For this review, take the finished solid that the model builds, in its own axes (mm). Face numbers are marked on the shaded views. A direction names the side the tool comes from. Round coordinates to 2 decimals unless told otherwise and drop trailing zeros. Order: outer loops, then holes, each group sorted by start corner. A loop starts at its lowest first (then second) coordinate and runs counter-clockwise, first axis right, second up. Notation, with made-up numbers: (77.5, -18) - (81.5, -18) arc R29 cw to (81.5, 13) - close; hole circle Ø3 at (32, -1). An arc over 180 degrees is marked (long way). One line per item, written item: value.
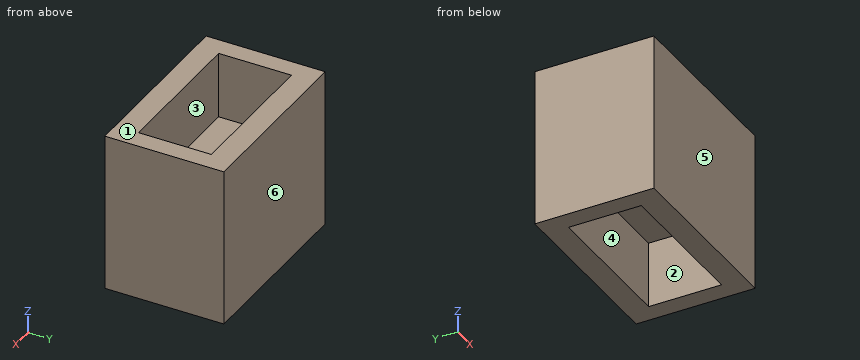
Autodesk Inventor part; units mm, degrees
ref_plane "YZ Plane" through (0, 0, 0) normal (1, 0, 0) x (0, 1, 0)
ref_plane "XZ Plane" through (0, 0, 0) normal (0, 1, 0) x (-1, 0, 0)
ref_plane "XY Plane" through (0, 0, 0) normal (0, 0, 1) x (1, 0, 0)
sketch "Sketch5" plane through (0, 0, 0) normal (0, 0, 1) x (1, 0, 0)
  line L0 (0, 0) -> (-13.9, 0)
  line L1 (-13.9, 0) -> (-13.9, 9)
  line L2 (-13.9, 9) -> (0, 9)
  line L3 (0, 9) -> (0, 0)
  line L4 (-2, 2) -> (-11.9, 2)
  line L5 (-11.9, 2) -> (-11.9, 7)
  line L6 (-11.9, 7) -> (-2, 7)
  line L7 (-2, 7) -> (-2, 2)
  dimension "d67" = 13.9
  dimension "d68" = 9
  dimension "d69" = 9.9
  dimension "d70" = 5
extrude "Extrusion8" add sketch "Sketch5" along normal blind 12 contours L0 L1 L2 L3 | L4 L5 L6 L7
sketch "Sketch10" plane through (0, 0, 12) normal (0, 0, 1) x (1, 0, 0)
  line L0 (-1.45, 1.75) -> (-12.45, 1.75)
  line L1 (-12.45, 1.75) -> (-12.45, 7.25)
  line L2 (-12.45, 7.25) -> (-1.45, 7.25)
  line L3 (-1.45, 7.25) -> (-1.45, 1.75)
  point P0 (0, 0)
  dimension "d99" = 11
  dimension "d100" = 5.5
sketch "Sketch11" plane through (0, 0, 0) normal (0, 0, -1) x (-1, 0, 0)
  line L0 (1.45, 1.75) -> (12.45, 1.75)
  line L1 (12.45, 1.75) -> (12.45, 7.25)
  line L2 (12.45, 7.25) -> (1.45, 7.25)
  line L3 (1.45, 7.25) -> (1.45, 1.75)
  point P0 (0, 0)
  dimension "d101" = 11
  dimension "d102" = 5.5
extrude "Extrusion16" cut sketch "Sketch10" against normal blind 5
extrude "Extrusion17" cut sketch "Sketch11" against normal blind 5
properties part number "Cube_Holder_SB_V1_(71mm)"
Item 1: Take a section at A-A (z = 10.25). Write out the cut boundary in (x, y), plus the area to 3 significant figures.
Returned:
outline: (-13.9, 0) - (0, 0) - (0, 9) - (-13.9, 9) - close; hole (-12.45, 1.75) - (-1.45, 1.75) - (-1.45, 7.25) - (-12.45, 7.25) - close
area: 64.6 mm^2
Item 2: The part is to be moulded in two halves that separate along Y. For the marked faces 4, 5 and 6, say which applies: +Y half, -Y half, draft (parallel to the pull), parting line (faces both ways), or undercut.
Returned:
face 4: undercut
face 5: -Y half
face 6: +Y half
Item 3: Take a section at B-B (x = -6). Write out the cut boundary in (y, z).
Returned:
outline: (0, 0) - (1.75, 0) - (1.75, 5) - (7.25, 5) - (7.25, 0) - (9, 0) - (9, 12) - (7.25, 12) - (7.25, 7) - (1.75, 7) - (1.75, 12) - (0, 12) - close
Item 4: Machinability: for the marked faces 1, 2 and 3, which of the approach directions +Z, -Z, +X, -X, +Y, -Y give a long, thin tool a straight path to every point of the face, cutting with its end or side? Answer none if there is none.
Returned:
face 1: +Z, +X, -X, +Y, -Y
face 2: -Z
face 3: +Z
Item 5: Take a section at C-C (y = 5.5). Write out the cut boundary in (x, z).
Returned:
outline: (-13.9, 0) - (-12.45, 0) - (-12.45, 5) - (-1.45, 5) - (-1.45, 0) - (0, 0) - (0, 12) - (-1.45, 12) - (-1.45, 7) - (-12.45, 7) - (-12.45, 12) - (-13.9, 12) - close
Item 6: For P1, Ø1.6, axis at x = -8.5, y = 4.5, coming from the -Z side, flat-tipped, find the tip position at first contact; note if it passes through.
Returned:
P1: z = 5
Item 7: Wall thickness on line 1 (X direction, y = 3.5, z = 4.25); line 2 (Y direction, x = -3.25, z = 10); line 3 (Z direction, x = -10.5, y = 6): over which ranges is each line inside the solid? List them lowest first.
Returned:
line 1: -13.9 to -12.45, -1.45 to 0
line 2: 0 to 1.75, 7.25 to 9
line 3: 5 to 7
